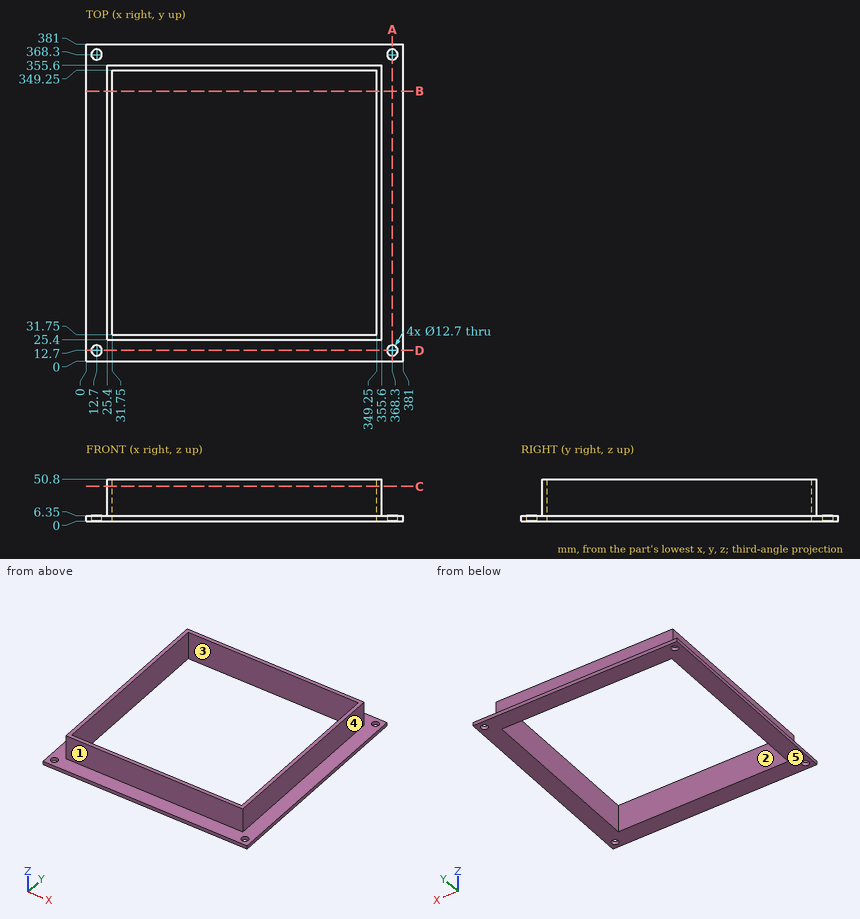
Design review of the part shown in the three views and the two pictorial views. Dimensions are in mm from the part's minimum x, y and z. A direction names the side the tool comes from. Round coordinates to 2 decimals unless told otherwise and drop trailing zeros. Loops run counter-clockwise (first coordinate to the right, second up) from the corner with the lowest first, then second, coordinate; pieces in that order, holes last. Notation, with made-up numbers: M 3.25,80 L 19.25,80 A17 ccw 19.25,90 Z; hole C 44.5,19.5 d2. An arc over 180 degrees is marked long. Answer as a JSON object with one key per item and string values.
Item 1: Clearance check with flat-ended pins moving along their axes: P1, Ø13.5, axis at y = 205.5, z = 24, coming from the -X side; P2, Ø4, axis at y = 81.5, z = 11.5, coming from the +X side; P3, Ø20.5, axis at x = 368.3, y = 368.3, coming from the +Z side. State where each tip first meets the part, or that it passes through.
Check sheet entries:
{"P1": "x = 25.4", "P2": "x = 355.6", "P3": "z = 6.35"}
Item 2: Tool access review of the marked faces 1 and 2: name each direction out of +Z, -Z, +X, -X, +Y, -Y from which nothing blocks a thin tool from reaching the whole face with its end or side.
Check sheet entries:
{"face 1": "+Z, +X, -X, -Y", "face 2": "+Z, -Z"}
Item 3: The part is to be moulded in two halves that separate along X. For the marked faces 3, 4 and 5, say which applies: +X half, -X half, draft (parallel to the pull), parting line (faces both ways), or undercut.
Check sheet entries:
{"face 3": "undercut", "face 4": "+X half", "face 5": "draft"}
Item 4: We need section A-A, the plane x = 368.3. State the section outline as (y, z) points, and give its area (3 significant figures).
Check sheet entries:
{"outline": "M 0,0 L 6.35,0 L 6.35,6.35 L 0,6.35 Z; M 19.05,0 L 361.95,0 L 361.95,6.35 L 19.05,6.35 Z; M 374.65,0 L 381,0 L 381,6.35 L 374.65,6.35 Z", "area": "2,260 mm2"}
Item 5: We need section B-B, the plane y = 324.5. State the section outline as (x, z) points, and give its area (3 significant figures).
Check sheet entries:
{"outline": "M 0,0 L 31.75,0 L 31.75,50.8 L 25.4,50.8 L 25.4,6.35 L 0,6.35 Z; M 349.25,0 L 381,0 L 381,6.35 L 355.6,6.35 L 355.6,50.8 L 349.25,50.8 Z", "area": "968 mm2"}
Item 6: We need section C-C, the plane z = 42. State the section outline as (x, y) points, and give its area (3 significant figures).
Check sheet entries:
{"outline": "M 25.4,25.4 L 355.6,25.4 L 355.6,355.6 L 25.4,355.6 Z; hole M 31.75,31.75 L 349.25,31.75 L 349.25,349.25 L 31.75,349.25 Z", "area": "8,230 mm2"}
Item 7: For line 1 along X through (y, z) = (12, 4); line 2 along X through (y, z) = (175.5, 33), list the stretches that pass through material, from the lowest coordinate up.
Check sheet entries:
{"line 1": "0 to 6.39, 19.01 to 361.99, 374.61 to 381", "line 2": "25.4 to 31.75, 349.25 to 355.6"}
